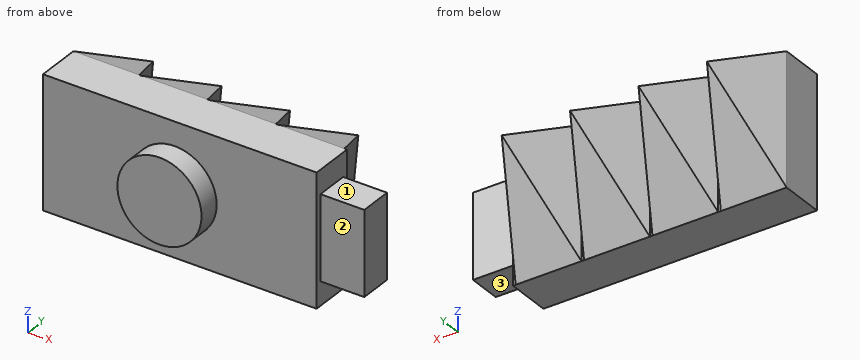
```python
from build123d import *

# Parameters (mm, degrees)
SKETCH1_W           = 19.05
SKETCH1_H           = 19.05
BOSS_EXTRUDE2_DEPTH = 6.35
SKETCH8_W           = 217.17
SKETCH8_H           = 38.1
BOSS_EXTRUDE4_DEPTH = 6.35
SKETCH8_5_W         = 217.17
SKETCH8_5_H         = 38.1
BOSS_EXTRUDE5_DEPTH = 6.4262
SKETCH9_W           = 19.05
SKETCH9_H           = 38.1
LPATTERN3_COUNT     = 11
LPATTERN3_PITCH     = 19.812
SKETCH15_R          = 12.192
BOSS_EXTRUDE6_DEPTH = 6.35
SKETCH16_W          = 57.265249545
SKETCH16_H          = 42.292481859
CUT_EXTRUDE1_DEPTH  = 137.922
SKETCH17_W          = 24.384
SKETCH17_H          = 9.5504
BOSS_EXTRUDE7_DEPTH = 12.7


with BuildPart() as part:
    # Sketch1 → Boss-Extrude2 (new body)
    with BuildSketch(Plane(origin=(0, 0, 0), x_dir=(1, 0, 0), z_dir=(0, 1, 0))):
        with Locations((9.525, -9.525)):
            Rectangle(SKETCH1_W, SKETCH1_H)
    extrude(amount=BOSS_EXTRUDE2_DEPTH)

    # Sketch8 → Boss-Extrude4 (add)
    with BuildSketch(Plane(origin=(0, 0, 0), x_dir=(1, 0, 0), z_dir=(0, 1, 0))):
        with Locations((108.585, -9.525)):
            Rectangle(SKETCH8_W, SKETCH8_H)
    extrude(amount=BOSS_EXTRUDE4_DEPTH)

    # Sketch8<5> → Boss-Extrude5 (add)
    with BuildSketch(Plane(origin=(0, 0, 0), x_dir=(1, 0, 0), z_dir=(0, 1, 0))):
        with Locations((108.585, -9.525)):
            Rectangle(SKETCH8_5_W, SKETCH8_5_H)
    extrude(amount=-BOSS_EXTRUDE5_DEPTH)

    # Sketch9 → Loft3 section 0
    with BuildSketch(Plane(origin=(0, 6.35, 0), x_dir=(1, 0, 0), z_dir=(0, 1, 0)), mode=Mode.PRIVATE) as loft3_s0:
        with Locations((9.525, -9.525)):
            Rectangle(SKETCH9_W, SKETCH9_H)
    loft3 = loft([loft3_s0.sketch, Vertex(9.525, 26.0731, 19.05)])

    # LPattern3: Loft3 ×11
    with Locations(*[(i * LPATTERN3_PITCH, 0, 0) for i in range(1, LPATTERN3_COUNT)]):
        add(loft3)

    # Sketch15 → Boss-Extrude6 (add)
    with BuildSketch(Plane.XZ.offset(6.4262)):
        with Locations((179.07, 9.525)):
            Circle(SKETCH15_R)
        with Locations((38.1, 9.525)):
            Circle(SKETCH15_R)
        with Locations((108.585, 9.525)):
            Circle(SKETCH15_R)
    extrude(amount=BOSS_EXTRUDE6_DEPTH)

    # Sketch16 → Cut-Extrude1 (cut)
    with BuildSketch(Plane(origin=(217.17, 0, 0), x_dir=(0, 0, -1), z_dir=(1, 0, 0))):
        with Locations((-10.111619629, 6.16028271)):
            Rectangle(SKETCH16_W, SKETCH16_H)
    extrude(amount=-CUT_EXTRUDE1_DEPTH, mode=Mode.SUBTRACT)

    # Sketch17 → Boss-Extrude7 (add)
    with BuildSketch(Plane(origin=(79.248, 0, 0), x_dir=(0, 0, -1), z_dir=(1, 0, 0))):
        with Locations((-9.525, -0.0381)):
            Rectangle(SKETCH17_W, SKETCH17_H)
    extrude(amount=BOSS_EXTRUDE7_DEPTH)


solid = part.part
```
Model file for the job. Use its own axes, mm. Face numbers are marked on the shaded views. A direction names the side the tool comes from. Coordinates: 2 decimals unless noted, no trailing zeros. Loops run counter-clockwise (first coordinate to the right, second up) from the corner with the lowest first, then second, coordinate; pieces in that order, holes last. Notation, with made-up numbers: (51.5, 8) -> (61.5, 8) arc R11 ccw to (61.5, 21) -> close; hole circle Ø6 at (-8, 44.5). An arc over 180 degrees is marked (long way). Answer as a JSON object with one key per item and string values.
Q1. Cut at C-C (x = 37). List the corners of the cut face in (y, z) (3 decimals), and give its area (3 significant figures).
Report:
{"outline": "(-12.776, -2.617) -> (-6.426, -2.617) -> (-6.426, -9.525) -> (6.35, -9.525) -> (10.206, -3.939) -> (10.206, 26.713) -> (6.35, 28.575) -> (-6.426, 28.575) -> (-6.426, 21.667) -> (-12.776, 21.667) -> close", "area": "774 mm2"}
Q2. Cut at A-A (y = 19). List the corners of the cut face in (x, z), and give its area (3 significant figures).
Report:
{"outline": "(6.11, 8.8) -> (12.94, 8.8) -> (12.94, 22.47) -> (6.11, 22.47) -> close; (25.92, 8.8) -> (32.75, 8.8) -> (32.75, 22.47) -> (25.92, 22.47) -> close; (45.73, 8.8) -> (52.56, 8.8) -> (52.56, 22.47) -> (45.73, 22.47) -> close; (65.55, 8.8) -> (72.38, 8.8) -> (72.38, 22.47) -> (65.55, 22.47) -> close", "area": "373 mm2"}
Q3. Cut at B-B (y = -1). List the corners of the cut face in (x, z) (3 decimals).
Report:
{"outline": "(0, -9.525) -> (79.248, -9.525) -> (79.248, -2.667) -> (91.948, -2.667) -> (91.948, 21.717) -> (79.248, 21.717) -> (79.248, 28.575) -> (0, 28.575) -> close"}
Q4. Probe probe 1 along X at (y, z) = (6, 2); probe 2 along X at (y, z) = (16.5, 15); probe 3 along X at (y, z) = (14, 10). List the from-to ranges inside material, lowest first.
Report:
{"probe 1": "x = 0 to 79.25", "probe 2": "x = 4.9 to 14.15, 24.71 to 33.96, 44.53 to 53.77, 64.34 to 73.58", "probe 3": "x = 3.69 to 15.36, 23.51 to 35.17, 43.32 to 54.98, 63.13 to 74.79"}
Q5. Cut at D-D (z = 16.5). List the corners of the cut face in (x, y) (3 decimals).
Report:
{"outline": "(0, -6.426) -> (28.1, -6.426) -> (28.1, -12.776) -> (48.1, -12.776) -> (48.1, -6.426) -> (79.248, -6.426) -> (79.248, -4.813) -> (91.948, -4.813) -> (91.948, 4.737) -> (79.248, 4.737) -> (79.248, 6.35) -> (78.486, 6.35) -> (69.811, 24.313) -> (68.111, 24.313) -> (59.436, 6.35) -> (58.674, 6.35) -> (49.999, 24.313) -> (48.299, 24.313) -> (39.624, 6.35) -> (38.862, 6.35) -> (30.187, 24.313) -> (28.487, 24.313) -> (19.812, 6.35) -> (19.05, 6.35) -> (10.375, 24.313) -> (8.675, 24.313) -> (0, 6.35) -> close"}
Q6. Flat gauge pins, fed straight in: P1, Ø7.5, axis at x = 86, y = -1, coming from the +Z side; P2, Ø10.5, axis at x = 85, y = -2.5, coming from the -Z side; P3, Ø8, axis at y = 10, z = 9, coming from the +X side. Where does each tip first touch, or does it go through?
Report:
{"P1": "stops at z = 21.72", "P2": "stops at z = -2.67", "P3": "stops at x = 79.25"}
Q7. 3-axis set-ups, long thin cutter, end or side, ignore diameter. For the marked faces 1, 2 and 3: which of +Z, -Z, +X, -X, +Y, -Y reach the whole face in a straight line?
Report:
{"face 1": "+Z, +X, +Y, -Y", "face 2": "+Z, -Z, +X, -Y", "face 3": "-Z, +X, +Y, -Y"}
